Check sheet for the drawn part. Datum: minimum x, y, z corner. Units: mm. Round coordinates to 2 decimals unless told otherwise and drop trailing zeros. Loops run counter-clockwise (first coordinate to the right, second up) from the corner with the lowest first, then second, coordinate; pieces in that order, holes last. Notation, with made-up numbers: (21.25, 48.5) -> (72.25, 48.5) arc R24 ccw to (72.25, 63.5) -> close; hole circle Ø1 at (83, 68). An arc over 180 degrees is marked (long way). Write item = value, one per line. Start each with the question number.
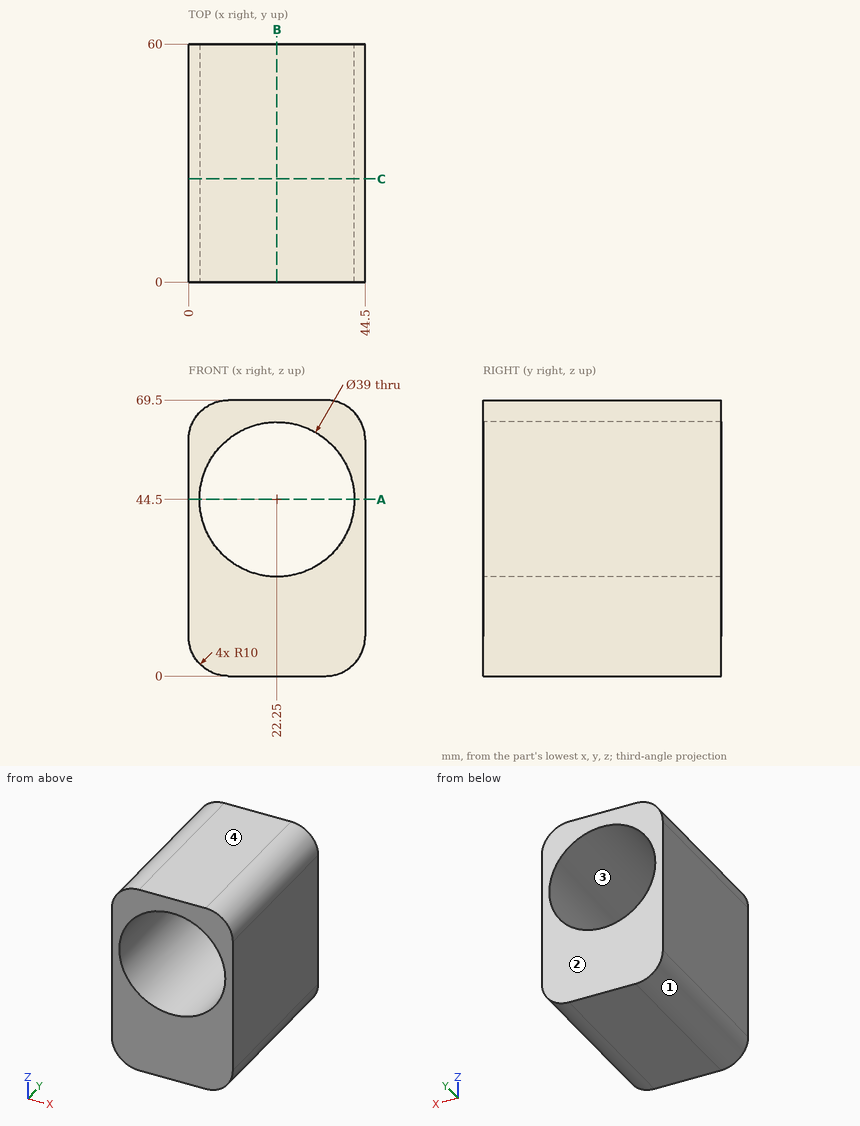
(1) Depth check by flat-ended pin: pin 1 Ø3 at (x, y) = (34.5, 23.5) entering from -Z. Enter the tip coordinate at first touch or a pass-through.
(2) Section check C-C on y = 26. Enter the section's corners in (x, z), then the cut area to 3 significant figures.
(3) Scan lines: line 1 (X direction, y = 16, z = 44); line 2 (Z direction, x = 22.25, y = 24.5); line 3 (Z direction, x = 40, y = 13.5). Record each from-to range of solid material in increasing order. Write a range as [from, to].
(4) Draft check along Z on the marked faces 1, 2, 3 and 4. Enter one of: +Z half, -Z half, draft (parallel to the pull), parting line (faces both ways), or undercut.
(5) Section check B-B on x = 22.25. Enter the section's corners in (y, z).
(6) Section check A-A on z = 44.5. Enter the section's corners in (x, y), then the cut area to 3 significant figures.
Computed values:
q1.pin_1 = 0
q2.outline = (0, 10) arc R10 ccw to (10, 0) -> (34.5, 0) arc R10 ccw to (44.5, 10) -> (44.5, 59.5) arc R10 ccw to (34.5, 69.5) -> (10, 69.5) arc R10 ccw to (0, 59.5) -> close; hole circle Ø39 at (22.25, 44.5)
q2.area = 1,810 mm²
q3.line_1 = [0, 2.76], [41.74, 44.5]
q3.line_2 = [0, 25], [64, 69.5]
q3.line_3 = [1.65, 36.43], [52.57, 67.85]
q4.face_1 = -Z half
q4.face_2 = draft
q4.face_3 = undercut
q4.face_4 = +Z half
q5.outline = (0, 0) -> (60, 0) -> (60, 25) -> (0, 25) -> close; (0, 64) -> (60, 64) -> (60, 69.5) -> (0, 69.5) -> close
q6.outline = (0, 0) -> (2.75, 0) -> (2.75, 60) -> (0, 60) -> close; (41.75, 0) -> (44.5, 0) -> (44.5, 60) -> (41.75, 60) -> close
q6.area = 330 mm²
